Here's how the part is built. I have some questions about the finished solid (model axes, mm). Face numbers are marked on the shaded views. A direction names the side the tool comes from. Coordinates: 2 decimals unless noted, no trailing zeros. Loops run counter-clockwise (first coordinate to the right, second up) from the corner with the lowest first, then second, coordinate; pieces in that order, holes last. Notation, with made-up numbers: M -4,27 L 5,27 A6 cw 5,32 Z; hole C -1.5,81.25 d2. An arc over 180 degrees is marked long. Use one line per item in the form item = value. Start each with the question number.
(1) Imagine slicing it at C-C, the plane z = 10.5. Please give me the cut outline in (x, y).
(2) On a 3-axis mill with a long thin cutter (end or side, diameter ignored), from which of +Z, -Z, +X, -X, +Y, -Y can I reach the whole of each face in a straight line? I mean the marked faces 5 and 6. Say none if no direction works.
(3) Please list where these lines run through material, in increasing order: L1, parallel to X at y = 2, z = 42; L2, parallel to Y at x = -27.5, z = 40.5; L3, parallel to X at y = 6.5, z = 14.
(4) Imagine slicing it at A-A, the plane y = 0. Please give me the cut outline in (x, z), and give its area (3 significant figures).
(5) Thinking about a two-plate mould opening in X: for the marked faces 1, 2, 3 and 4, which applies, +X half, -X half, draft (parallel to the pull), parting line (faces both ways), or undercut?
(6) Imagine slicing it at B-B, the plane z = 54. Please give me the cut outline in (x, y), and give its area (3 significant figures).
(7) Imagine slicing it at D-D, the plane x = -50.5. Please give me the cut outline in (y, z).
(8) Will these pins go through, and if not, where does the flat tip stop? P1, Ø18, axis at x = 44.75, y = 0, coming from the +Z side; P2, Ø2, axis at x = 41, z = 56, coming from the -Y side.
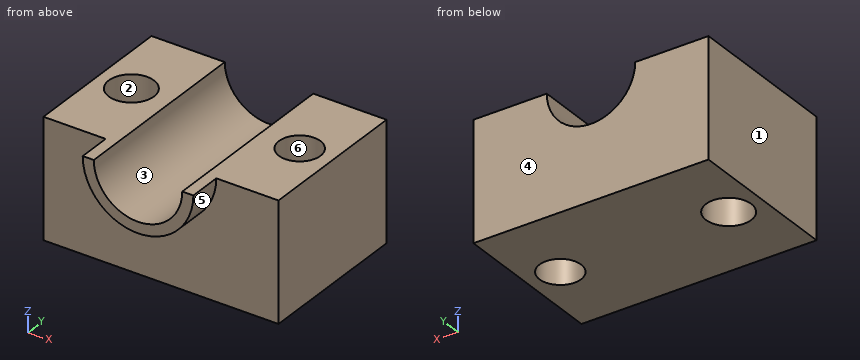
```python
from build123d import *

# Parameters (mm, degrees)
F0_W     = 125.7711164653
F0_H     = 83.7514773011
F0_R     = 12.1092368637
F0_R_2   = 11.1364451926
F1_DEPTH = 63.5
F3_DEPTH = 17.78
F4_DEPTH = 98.044


with BuildPart() as f1:
    # F0 (on Top) → F1 (new body)
    with BuildSketch(Plane.XY):
        with Locations((-0.5756113678, 0)):
            Rectangle(F0_W, F0_H)
        with Locations((-45.3294068575, 0)):
            Circle(F0_R, mode=Mode.SUBTRACT)
        with Locations((44.7537973523, 0)):
            Circle(F0_R_2, mode=Mode.SUBTRACT)
    extrude(amount=F1_DEPTH)

    # F2 (on face) → F3 (join)
    with BuildSketch(Plane.XZ.offset(41.8757386506)):
        with BuildLine():
            Line((29.0334055844, 63.5), (23.0987426611, 63.5))
            ThreePointArc((23.0987426611, 63.5), (-0.5756113678, 39.8256459711), (-24.2499653967, 63.5))
            Line((-24.2499653967, 63.5), (-30.1846283201, 63.5))
            ThreePointArc((-30.1846283201, 63.5), (-0.5756113678, 33.8909830478), (29.0334055844, 63.5))
        make_face()
    extrude(amount=F3_DEPTH)

    # F4 (cut): a face of the model
    f4_faces = [f1.faces().sort_by_distance(p)[0] for p in [
        (-0.5756113678, -41.8757386506, 53.4522920848),
    ]]
    extrude(f4_faces, amount=-F4_DEPTH, mode=Mode.SUBTRACT)


solid = f1.part
```
Answer:
q1.outline = M -63.46,-41.88 L 62.31,-41.88 L 62.31,41.88 L -63.46,41.88 Z; hole C -45.33,0 d24.22; hole C 44.75,0 d22.27
q2.face_5 = -Z, -Y
q2.face_6 = +Z, -Z
q3.L1 = -63.46 to -57.27, -33.39 to -10.49, 9.34 to 33.8, 55.71 to 62.31
q3.L2 = -41.88 to 41.88
q3.L3 = -63.46 to -55.55, -35.11 to 35.71, 53.8 to 62.31
q4.outline = M -63.46,0 L -57.44,0 L -57.44,63.5 L -63.46,63.5 Z; M -33.22,0 L 33.62,0 L 33.62,63.5 L 23.1,63.5 A23.67 cw -24.25,63.5 L -33.22,63.5 Z; M 55.89,0 L 62.31,0 L 62.31,63.5 L 55.89,63.5 Z
q4.area = 4,150 mm²
q5.face_1 = -X half
q5.face_2 = undercut
q5.face_3 = undercut
q5.face_4 = draft
q6.outline = M -63.46,-41.88 L -28.62,-41.88 L -28.62,-59.66 L -22.26,-59.66 L -22.26,41.88 L -63.46,41.88 Z; M 21.11,-59.66 L 27.47,-59.66 L 27.47,-41.88 L 62.31,-41.88 L 62.31,41.88 L 21.11,41.88 Z; hole C -45.33,0 d24.22; hole C 44.75,0 d22.27
q6.area = 6,280 mm²
q7.outline = M -41.88,0 L -10.95,0 L -10.95,63.5 L -41.88,63.5 Z; M 10.95,0 L 41.88,0 L 41.88,63.5 L 10.95,63.5 Z
q8.P1 = through
q8.P2 = -41.88
